Verification items for the finished model (mm, model axes). Coordinates: 2 decimals unless noted, no trailing zeros. Write each loop counter-clockwise with the first axis right and the second up, starting at its lowest first coordinate (ties: lowest second). Pieces come first, ordered by that corner, then holes. Notation, with made-up numbers: (8.5, 26) -> (43.5, 26) arc R30 ccw to (43.5, 54) -> close; hole circle Ø5 at (48, -35). An arc over 180 degrees is marked (long way). Answer in a Markdown table with one row per item.
Autodesk Inventor part; units mm, degrees
ref_plane "YZ Plane" through (0, 0, 0) normal (1, 0, 0) x (0, 1, 0)
ref_plane "XZ Plane" through (0, 0, 0) normal (0, 1, 0) x (-1, 0, 0)
ref_plane "XY Plane" through (0, 0, 0) normal (0, 0, 1) x (1, 0, 0)
sketch "Sketch1" plane through (0, 0, 0) normal (0, 0, 1) x (1, 0, 0)
  line L0 (0, 0) -> (190.5, 0)
  line L1 (190.5, 0) -> (190.5, 80)
  line L2 (190.5, 80) -> (0, 80)
  line L3 (0, 80) -> (0, 0)
  dimension "d0" = 80
  dimension "d1" = 190.5
extrude "Extrusion1" add sketch "Sketch1" along normal blind 7.62
sketch "Sketch2" plane through (0, 0, 7.62) normal (0, 0, 1) x (1, 0, 0)
  line L0 (45.25, 15) -> (145.25, 15) construction
  line L1 (145.25, 15) -> (145.25, 65) construction
  line L2 (145.25, 65) -> (45.25, 65) construction
  line L3 (45.25, 65) -> (45.25, 15) construction
  line L4 (190.5, 80) -> (0, 80) construction
  line L5 (190.5, 0) -> (190.5, 80) construction
  circle A0 centre (45.25, 65) radius 4
  circle A1 centre (145.25, 65) radius 4
  circle A2 centre (45.25, 15) radius 4
  circle A3 centre (145.25, 15) radius 4
  point P0 (0, 0)
  point P1 (95.25, 65)
  point P2 (95.25, 80)
  point P3 (145.25, 40)
  point P4 (190.5, 40)
  dimension "d4" = 100
  dimension "d5" = 50
  dimension "d6" = 8
extrude "Extrusion2" cut sketch "Sketch2" against normal up to surface (7.62 mm away)
sketch "Sketch3" plane through (0, 0, 7.62) normal (0, 0, 1) x (1, 0, 0)
  line L0 (7.75, 20) -> (62.75, 20) construction
  line L1 (62.75, 20) -> (62.75, 60) construction
  line L2 (62.75, 60) -> (7.75, 60) construction
  line L3 (7.75, 60) -> (7.75, 20) construction
  circle A0 centre (7.75, 60) radius 2.5
  circle A1 centre (62.75, 60) radius 2.5
  circle A2 centre (7.75, 20) radius 2.5
  circle A3 centre (62.75, 20) radius 2.5
  line L4 (190.5, 80) -> (0, 80) construction
  line L5 (95.25, 80) -> (95.25, 0)
  line L6 (0, 0) -> (190.5, 0) construction
  circle A4 centre (182.75, 60) radius 2.5
  circle A5 centre (127.75, 60) radius 2.5
  circle A6 centre (182.75, 20) radius 2.5
  circle A7 centre (127.75, 20) radius 2.5
  point P0 (62.75, 40)
  point P1 (35.25, 60)
  point P2 (95.25, 40)
  dimension "d9" = 5
  dimension "d10" = 55
  dimension "d11" = 40
  dimension "d12" = 60
extrude "Extrusion3" cut sketch "Sketch3" against normal up to surface (7.62 mm away)
sketch "Sketch4" plane through (0, 0, 7.62) normal (0, 0, 1) x (1, 0, 0)
  line L0 (77.75, 50) -> (112.75, 50) construction
  line L1 (112.75, 50) -> (112.75, 74) construction
  line L2 (112.75, 74) -> (77.75, 74) construction
  line L3 (77.75, 74) -> (77.75, 50) construction
  circle A0 centre (112.75, 50) radius 2.5
  circle A1 centre (112.75, 74) radius 2.5
  circle A2 centre (77.75, 74) radius 2.5
  circle A3 centre (77.75, 50) radius 2.5
  line L4 (190.5, 80) -> (0, 80) construction
  line L5 (190.5, 0) -> (190.5, 80) construction
  point P0 (0, 0)
  point P1 (95.25, 50)
  point P2 (95.25, 80)
  point P3 (190.5, 40)
  point P4 (112.75, 62)
  dimension "d15" = 5
  dimension "d16" = 35
  dimension "d17" = 24
  dimension "d18" = 6
extrude "Extrusion4" cut sketch "Sketch4" against normal up to surface (7.62 mm away)
properties part number "Spindle_Mounting_Plate"
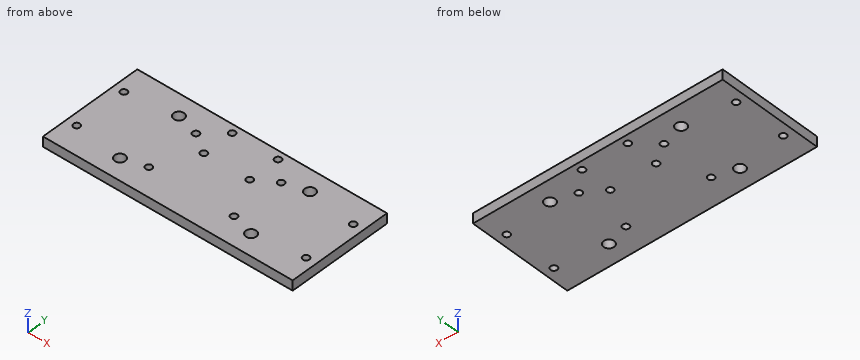
1. Thickness scan on line 1 (Y direction, x = 145.25, z = 2.75); line 2 (X direction, y = 12, z = 2.75); line 3 (Y direction, x = 64.5, z = 6.5). Record the ranges inside material, lowest first. Write a range as from..to.
Geometry says:
| item | result |
|---|---|
| line 1 | 0..11, 19..61, 69..80 |
| line 2 | 0..42.6, 47.9..142.6, 147.9..190.5 |
| line 3 | 0..18.21, 21.79..58.21, 61.79..80 |
2. Depth check by flat-ended pin: P1, Ø5, axis at x = 45.25, y = 15, coming from the +Z side. Enter the tip coordinate at first touch or a pass-through.
Geometry says:
| item | result |
|---|---|
| P1 | through |
3. Section check C-C, the plane z = 1.5. State how many separate pieces and enclosed holes the cut face has, plus the area to 3 significant figures.
Geometry says:
| item | result |
|---|---|
| separate pieces | 1 |
| enclosed holes | 16 |
| area | 14,800 mm^2 |
4. Section check A-A, the plane x = 145.25. Record the boundary of the cut face in (y, z).
Geometry says:
| item | result |
|---|---|
| outline | (0, 0) -> (11, 0) -> (11, 7.62) -> (0, 7.62) -> close; (19, 0) -> (61, 0) -> (61, 7.62) -> (19, 7.62) -> close; (69, 0) -> (80, 0) -> (80, 7.62) -> (69, 7.62) -> close |
5. Section check B-B, the plane y = 15. Record the boundary of the cut face in (x, z), plus the area to 3 significant figures.
Geometry says:
| item | result |
|---|---|
| outline | (0, 0) -> (41.25, 0) -> (41.25, 7.62) -> (0, 7.62) -> close; (49.25, 0) -> (141.25, 0) -> (141.25, 7.62) -> (49.25, 7.62) -> close; (149.25, 0) -> (190.5, 0) -> (190.5, 7.62) -> (149.25, 7.62) -> close |
| area | 1,330 mm^2 |
